```python
from build123d import *

# Parameters (mm, degrees)
F0_W      = 67.0393481851
F0_H      = 127.374753356
F1_DEPTH  = 3.55
F2_T      = -2.54
F3_R      = 5.08
F6_DEPTH  = 12.7
F7_W      = 26.815738529
F7_H      = 6.7039346322
F8_DEPTH  = 12.7
F10_DEPTH = 12.5
F12_DEPTH = 12.5


with BuildPart() as f1:
    # F0 (on Front) → F1 (new body, symmetric)
    with BuildSketch(Plane.XZ):
        Rectangle(F0_W, F0_H)
    extrude(amount=F1_DEPTH, both=True)

    # F2
    f2_openings = [f1.faces().sort_by_distance(p)[0] for p in [
        (0, -3.55, 0),
    ]]
    offset(amount=F2_T, openings=f2_openings)

    # F3
    f3_edges = [f1.edges().sort_by_distance(p)[0] for p in [
        (33.519674, 0, -63.687377),
        (-33.519674, 0, -63.687377),
        (-33.519674, 0, 63.687377),
        (33.519674, 0, 63.687377),
    ]]
    fillet(f3_edges, radius=F3_R)

    # F5 (on face) → F6 (cut, symmetric)
    with BuildSketch(Plane.XZ.offset(-1.01)):
        with BuildLine():
            add(Edge.make_bspline(
                [(24.4839340448, 52.3198395967), (24.4839340448, 60.4477757444), (8.7442607619, 56.3838076706), (-6.9954125211, 52.3198395967), (8.7442607619, 48.2558715229), (24.4839340448, 44.1919034491), (24.4839340448, 52.3198395967)],
                knots=[0, 0, 0, 2.0943951024, 2.0943951024, 4.1887902048, 4.1887902048, 6.2831853072, 6.2831853072, 6.2831853072], degree=2, weights=[1, 0.5, 1, 0.5, 1, 0.5, 1]))
        make_face()
    extrude(amount=F6_DEPTH, both=True, mode=Mode.SUBTRACT)

    # F7 (on face) → F8 (cut, symmetric)
    with BuildSketch(Plane(origin=(0, 0, -63.687376678), x_dir=(1, 0, 0), z_dir=(0, 0, -1))):
        Rectangle(F7_W, F7_H)
    extrude(amount=F8_DEPTH, both=True, mode=Mode.SUBTRACT)

    # F9 (on face) → F10 (cut, symmetric)
    with BuildSketch(Plane(origin=(-33.5196740925, 0, 0), x_dir=(0, -1, 0), z_dir=(-1, 0, 0))):
        with BuildLine():
            add(Edge.make_bspline(
                [(0, 28.9168681979), (4.0015380048, 28.9168681979), (2.0007690024, 35.6668681979), (0, 42.4168681979), (-2.0007690024, 35.6668681979), (-4.0015380048, 28.9168681979), (0, 28.9168681979)],
                knots=[0, 0, 0, 2.0943951024, 2.0943951024, 4.1887902048, 4.1887902048, 6.2831853072, 6.2831853072, 6.2831853072], degree=2, weights=[1, 0.5, 1, 0.5, 1, 0.5, 1]))
        make_face()
    extrude(amount=F10_DEPTH, both=True, mode=Mode.SUBTRACT)

    # F11 (on face) → F12 (cut, symmetric)
    with BuildSketch(Plane(origin=(-33.5196740925, 0, 0), x_dir=(0, -1, 0), z_dir=(-1, 0, 0))):
        with BuildLine():
            add(Edge.make_bspline(
                [(0, 28.9168681979), (1.2599189299, 28.9168681979), (1.9422093652, 30.9799598491)],
                knots=[0, 0, 0, 1.0030560238, 1.0030560238, 1.0030560238], degree=2, weights=[1, 0.7605380134, 0.7504441989]))
            add(Edge.make_bspline(
                [(1.9422093652, 30.9799598491), (0, 35.0307743016), (-1.9422093652, 30.9799598491)],
                knots=[2.3582521763, 2.3582521763, 2.3582521763, 3.9249331309, 3.9249331309, 3.9249331309], degree=2, weights=[1, 0.708560287, 1]))
            add(Edge.make_bspline(
                [(-1.9422093652, 30.9799598491), (-1.2599189299, 28.9168681979), (0, 28.9168681979)],
                knots=[5.2801292834, 5.2801292834, 5.2801292834, 6.2831853072, 6.2831853072, 6.2831853072], degree=2, weights=[0.7504441989, 0.7605380134, 1]))
        make_face()
        with BuildLine():
            add(Edge.make_bspline(
                [(-1.9422093652, 30.9799598491), (-6.6641891215, 21.131452173), (0, 21.131452173)],
                knots=[3.9249331309, 3.9249331309, 3.9249331309, 6.2831853072, 6.2831853072, 6.2831853072], degree=2, weights=[1, 0.381732703, 1]))
            add(Edge.make_bspline(
                [(0, 21.131452173), (6.6641891215, 21.131452173), (1.9422093652, 30.9799598491)],
                knots=[0, 0, 0, 2.3582521763, 2.3582521763, 2.3582521763], degree=2, weights=[1, 0.381732703, 1]))
            add(Edge.make_bspline(
                [(0, 28.9168681979), (1.2599189299, 28.9168681979), (1.9422093652, 30.9799598491)],
                knots=[0, 0, 0, 1.0030560238, 1.0030560238, 1.0030560238], degree=2, weights=[1, 0.7605380134, 0.7504441989]))
            add(Edge.make_bspline(
                [(-1.9422093652, 30.9799598491), (-1.2599189299, 28.9168681979), (0, 28.9168681979)],
                knots=[5.2801292834, 5.2801292834, 5.2801292834, 6.2831853072, 6.2831853072, 6.2831853072], degree=2, weights=[0.7504441989, 0.7605380134, 1]))
        make_face()
    extrude(amount=F12_DEPTH, both=True, mode=Mode.SUBTRACT)


solid = f1.part
```
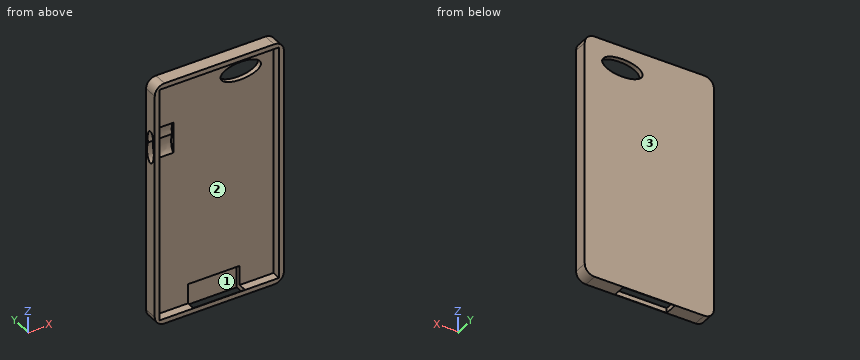
CAD build for the part. Positions are in the model's coordinates, mm. Face numbers are marked on the shaded views. Give positions to 0.01 mm unless a question says otherwise; leave off trailing zeros. Write each loop counter-clockwise with the first axis right and the second up, starting at its lowest first coordinate (ties: lowest second). Pieces come first, ordered by that corner, then holes. Notation, with made-up numbers: M -40,21.25 L -16,21.25 A20 cw -16,25.25 Z; hole C 88.5,65.5 d7. An arc over 180 degrees is marked long. Return JSON: item names as keys, results as strings. Group by question number.
(1) Band-saw the part on B-B (z = -21.5). Give the cut face in (x, y).
(2) Band-saw the part on A-A (x = -8). Give the cut face in (y, z), and give its area (3 significant figures).
(3) Mould opens along X. For the marked faces 1, 2 and 3 say: pulls with the +X half, pulls with the -X half, needs draft (parallel to the pull), parting line crosses it, or undercut.
(4) Flat gauge pins, fed straight in: pin 1 Ø0.9 at (y, z) = (1.5, 31.5) entering from -X; pin 2 Ø2 at (x, z) = (1, 41.5) entering from -Y; pin 3 Ø1.2 at (x, y) = (-6.5, 2.5) entering from -Z. Where does each tip first touch, or does it go through?
(5) Drill centre lines: L1, parallel to X at y = -2, z = 57.5; L2, parallel to Z at x = -23, y = -1; L3, parallel to Z at x = 13.5, y = 3.25. Where is each one in solid material? Low to high. Write a range as [from, to].
Entries:
{
 "1": {"outline": "M -33.52,-3.55 L -30.98,-3.55 L -30.98,1.01 L 30.98,1.01 L 30.98,-3.55 L 33.52,-3.55 L 33.52,3.55 L -33.52,3.55 Z"},
 "2": {"outline": "M -3.55,-63.69 L -3.35,-63.69 L -3.35,-61.15 L -3.55,-61.15 Z; M -3.55,61.15 L 1.01,61.15 L 1.01,-50.99 L 3.35,-50.99 L 3.35,-63.69 L 3.55,-63.69 L 3.55,63.69 L -3.55,63.69 Z", "area": "306 mm^2"},
 "3": {"face 1": "undercut", "face 2": "undercut", "face 3": "needs draft"},
 "4": {"pin 1": "stops at x = -21.02", "pin 2": "stops at y = 1.01", "pin 3": "stops at z = -50.99"},
 "5": {"L1": "x = [-33.52, -30.98], [30.98, 33.52]", "L2": "z = [-63.69, -61.15], [61.15, 63.69]", "L3": "z = [-63.69, 47.63], [57.01, 63.69]"}
}
